```python
from build123d import *

# Parameters (mm, degrees)
SKETCH1_R           = 8
SKETCH1_R_2         = 2.5
BOSS_EXTRUDE1_DEPTH = 26
SKETCH2_R           = 3.5
CUT_EXTRUDE1_DEPTH  = 10


with BuildPart() as part:
    # Sketch1 → Boss-Extrude1 (new body)
    with BuildSketch(Plane.XY):
        Circle(SKETCH1_R)
        Circle(SKETCH1_R_2, mode=Mode.SUBTRACT)
    extrude(amount=BOSS_EXTRUDE1_DEPTH)

    # Sketch2 → Cut-Extrude1 (cut)
    with BuildSketch(Plane.XY.offset(18)):
        Circle(SKETCH2_R)
    extrude(amount=-CUT_EXTRUDE1_DEPTH, mode=Mode.SUBTRACT)


solid = part.part
```
The model under review builds one solid part; all positions refer to its coordinate system, in mm. A direction names the side the tool comes from. Round coordinates to 2 decimals unless told otherwise and drop trailing zeros. Loops run counter-clockwise (first coordinate to the right, second up) from the corner with the lowest first, then second, coordinate; pieces in that order, holes last. Notation, with made-up numbers: (-30, 43.25) -> (15, 43.25) arc R27 cw to (15, 69.25) -> close; hole circle Ø6 at (-27.5, 13.25). An arc over 180 degrees is marked (long way). Answer in a Markdown table with one row per item.
1) Consider section A-A, the plane y = 0. Write out the cut boundary in (x, z), plus the area to 3 significant figures.
Taken from the geometry:
| item | result |
|---|---|
| outline | (-8, 0) -> (-2.5, 0) -> (-2.5, 8) -> (-3.5, 8) -> (-3.5, 18) -> (-2.5, 18) -> (-2.5, 26) -> (-8, 26) -> close; (2.5, 0) -> (8, 0) -> (8, 26) -> (2.5, 26) -> (2.5, 18) -> (3.5, 18) -> (3.5, 8) -> (2.5, 8) -> close |
| area | 266 mm² |
2) Wall thickness on line 1 along Y through (x, z) = (0, 11); line 2 along Y through (x, z) = (0, 2.25); line 3 along Z through (x, y) = (-0.5, 3): over which ranges is each line inside the solid? List them lowest first.
Taken from the geometry:
| item | result |
|---|---|
| line 1 | y = -8 to -3.5, 3.5 to 8 |
| line 2 | y = -8 to -2.5, 2.5 to 8 |
| line 3 | z = 0 to 8, 18 to 26 |
3) Draft analysis for pull direction X (two halves, no side actions). For faces 3 (the flat face through (2, -2, 18)), 4 (the flat face through (2, 2, 26)), 5 (the cylindrical face through (-1.73, -7.81, 12.82)), state which applies: pulls with the +X half, pulls with the -X half, needs draft (parallel to the pull), parting line crosses it, or undercut.
Taken from the geometry:
| item | result |
|---|---|
| face 3 | undercut |
| face 4 | needs draft |
| face 5 | parting line crosses it |
4) Consider section C-C, the plane z = 14. Write out the cut boundary in (x, y), plus the area to 3 significant figures.
Taken from the geometry:
| item | result |
|---|---|
| outline | circle Ø16 at (0, 0); hole circle Ø7 at (0, 0) |
| area | 163 mm² |
5) Tool access review of faces 1 (the cylindrical face through (3.233, -1.341, 13.07)), 2 (the flat face through (2, 2, 0)): name each direction out of +Z, -Z, +X, -X, +Y, -Y from which nothing blocks a thin tool from reaching the whole face with its end or side.
Taken from the geometry:
| item | result |
|---|---|
| face 1 | none |
| face 2 | -Z, +X, -X, +Y, -Y |
6) For pin 1 Ø4 at (x, y) = (0, 0) entering from -Z; pin 2 Ø1 at (x, z) = (-3, 18.5) entering from +Y; pin 3 Ø3 at (y, z) = (-6, 3) entering from +X; pin 4 Ø4 at (y, z) = (-5, 5.5) entering from +X, all flat-tipped, find the tip position at first contact; note any pin that passes through.
Taken from the geometry:
| item | result |
|---|---|
| pin 1 | passes through |
| pin 2 | stops at y = 7.6 |
| pin 3 | stops at x = 6.61 |
| pin 4 | stops at x = 7.42 |
7) Consider section D-D, the plane x = -4.5. Write out the cut boundary in (y, z).
Taken from the geometry:
| item | result |
|---|---|
| outline | (-6.61, 0) -> (6.61, 0) -> (6.61, 26) -> (-6.61, 26) -> close |
